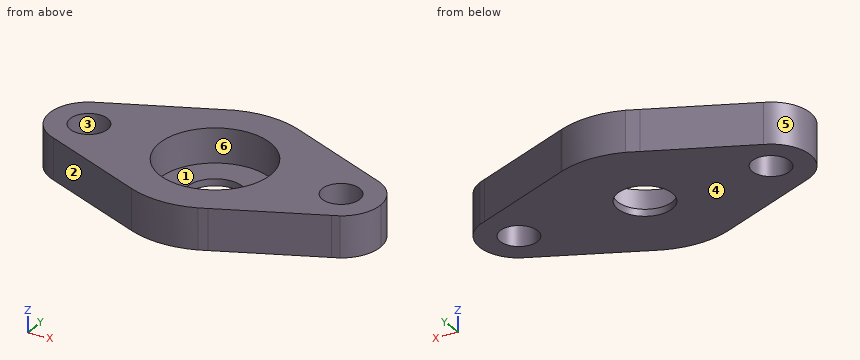
from build123d import *

# Parameters (mm, degrees)
F0_R     = 2.75
F0_R_2   = 4
F1_DEPTH = 6
F2_R     = 8.125
F2_R_2   = 4
F3_DEPTH = 5


# Not quite as in the source:
# - a feature names something its author has since deleted; it is built from what else it names


with BuildPart() as f1:
    # F0 (on Top) → F1 (new body)
    with BuildSketch(Plane.XY):
        with BuildLine():
            ThreePointArc((20.0822139412, 5.4502744952), (15.7589539647, 5.182392271), (12.8493150685, 1.9736013454))
            ThreePointArc((12.8493150685, 1.9736013454), (12.9622740268, 0.9896727008), (13, 0))
            ThreePointArc((13, 0), (12.9622740268, -0.9896727008), (12.8493150685, -1.9736013454))
            ThreePointArc((12.8493150685, -1.9736013454), (15.7262122641, -5.1665264409), (20.0130954241, -5.4730242577))
            Line((20.0130954241, -5.4730242577), (21.0412591059, -5.0270640143))
            ThreePointArc((21.0412591059, -5.0270640143), (23.2054131946, -2.9165699153), (24, 0))
            ThreePointArc((24, 0), (23.1883419046, 2.9453826972), (20.982511571, 5.0592371474))
            Line((20.982511571, 5.0592371474), (20.0822139412, 5.4502744952))
        make_face()
        with Locations((18.25, 0)):
            Circle(F0_R, mode=Mode.SUBTRACT)
        with BuildLine():
            Line((20.0822139412, 5.4502744952), (5.2758693561, 11.8812963323))
            ThreePointArc((5.2758693561, 11.8812963323), (10.328174214, 7.8948601891), (12.8493150685, 1.9736013454))
            ThreePointArc((12.8493150685, 1.9736013454), (15.7589539647, 5.182392271), (20.0822139412, 5.4502744952))
        make_face()
        with BuildLine():
            ThreePointArc((13, 0), (12.9622740268, 0.9896727008), (12.8493150685, 1.9736013454))
            ThreePointArc((12.8493150685, 1.9736013454), (12.5, 0), (12.8493150685, -1.9736013454))
            ThreePointArc((12.8493150685, -1.9736013454), (12.9622740268, -0.9896727008), (13, 0))
        make_face()
        with BuildLine():
            ThreePointArc((20.0130954241, -5.4730242577), (15.7262122641, -5.1665264409), (12.8493150685, -1.9736013454))
            ThreePointArc((12.8493150685, -1.9736013454), (10.4831727002, -7.6878534154), (5.7442785493, -11.6620437295))
            Line((5.7442785493, -11.6620437295), (20.0130954241, -5.4730242577))
        make_face()
        with BuildLine():
            Line((5.2758693561, 11.8812963323), (5.0818351063, 11.9655736157))
            ThreePointArc((5.0818351063, 11.9655736157), (0.4274688612, 12.9929700366), (-4.2843620194, 12.273721607))
            Line((-4.2843620194, 12.273721607), (-5.9821590265, 11.5418271249))
            ThreePointArc((-5.9821590265, 11.5418271249), (-10.5614317348, 7.5799841498), (-12.8493150685, 1.9736013454))
            ThreePointArc((-12.8493150685, 1.9736013454), (-12.588002192, 1.0021381252), (-12.5, 0))
            ThreePointArc((-12.5, 0), (-12.588002192, -1.0021381252), (-12.8493150685, -1.9736013454))
            ThreePointArc((-12.8493150685, -1.9736013454), (-10.2925346971, -7.9412675001), (-5.1687008476, -11.9283079918))
            ThreePointArc((-5.1687008476, -11.9283079918), (-0.3123803464, -12.9962463242), (4.589640736, -12.1628614197))
            Line((4.589640736, -12.1628614197), (5.7442785493, -11.6620437295))
            ThreePointArc((5.7442785493, -11.6620437295), (10.4831727002, -7.6878534154), (12.8493150685, -1.9736013454))
            ThreePointArc((12.8493150685, -1.9736013454), (12.5, 0), (12.8493150685, 1.9736013454))
            ThreePointArc((12.8493150685, 1.9736013454), (10.328174214, 7.8948601891), (5.2758693561, 11.8812963323))
        make_face()
        Circle(F0_R_2, mode=Mode.SUBTRACT)
        with BuildLine():
            ThreePointArc((-12.8493150685, -1.9736013454), (-13, 0), (-12.8493150685, 1.9736013454))
            ThreePointArc((-12.8493150685, 1.9736013454), (-15.8411768162, 5.2211177797), (-20.2535684755, 5.3896394466))
            ThreePointArc((-20.2535684755, 5.3896394466), (-23.9999641766, 0.020296977), (-20.2915681825, -5.3753603932))
            ThreePointArc((-20.2915681825, -5.3753603932), (-15.8596218943, -5.229588178), (-12.8493150685, -1.9736013454))
        make_face()
        with Locations((-18.25, 0)):
            Circle(F0_R, mode=Mode.SUBTRACT)
        with BuildLine():
            ThreePointArc((-12.5, 0), (-12.588002192, 1.0021381252), (-12.8493150685, 1.9736013454))
            ThreePointArc((-12.8493150685, 1.9736013454), (-13, 0), (-12.8493150685, -1.9736013454))
            ThreePointArc((-12.8493150685, -1.9736013454), (-12.588002192, -1.0021381252), (-12.5, 0))
        make_face()
        with BuildLine():
            ThreePointArc((-12.8493150685, 1.9736013454), (-10.5614317348, 7.5799841498), (-5.9821590265, 11.5418271249))
            Line((-5.9821590265, 11.5418271249), (-20.2535684755, 5.3896394466))
            ThreePointArc((-20.2535684755, 5.3896394466), (-15.8411768162, 5.2211177797), (-12.8493150685, 1.9736013454))
        make_face()
        with BuildLine():
            ThreePointArc((-5.1687008476, -11.9283079918), (-10.2925346971, -7.9412675001), (-12.8493150685, -1.9736013454))
            ThreePointArc((-12.8493150685, -1.9736013454), (-15.8596218943, -5.229588178), (-20.2915681825, -5.3753603932))
            Line((-20.2915681825, -5.3753603932), (-5.1687008476, -11.9283079918))
        make_face()
    extrude(amount=F1_DEPTH)

    # F2 (on face) → F3 (cut)
    with BuildSketch(Plane.XY.offset(6)):
        Circle(F2_R)
        Circle(F2_R_2, mode=Mode.SUBTRACT)
    extrude(amount=-F3_DEPTH, mode=Mode.SUBTRACT)


solid = f1.part
Geometry check sheet. Reference: the model listing, model coordinates, mm. Face numbers are marked on the shaded views. A direction names the side the tool comes from. Round coordinates to 2 decimals unless told otherwise and drop trailing zeros. Loops run counter-clockwise (first coordinate to the right, second up) from the corner with the lowest first, then second, coordinate; pieces in that order, holes last. Notation, with made-up numbers: (-28.5, 25) - (-17.5, 25) arc R31 ccw to (-17.5, 57) - close; hole circle Ø6 at (81, 63.25). An arc over 180 degrees is marked (long way). One line per question, with ' | ' between items. Start each with the question number.
1. Cross-section at C-C on y = 1.5. Record the cut outline in (x, z), then the cut area to 3 significant figures.
2. Cross-section at A-A on x = 0. Record the cut outline in (y, z) (3 decimals), then the cut area to 4 significant figures.
3. Tool access check on the marked faces 1 and 2. Record the directions out of +Z, -Z, +X, -X, +Y, -Y that give a thin tool (end or side, any length) a straight path to the whole face; none if there is none.
4. Draft check along X on the marked faces 3, 4, 5 and 6. Enter one of: released by +X, released by -X, zero draft, split by the parting line, or undercut.
5. Depth check by flat-ended pin: pin 1 (2 mm diameter, centred on x = 14.5, z = 1.5, fed in from -Y); pin 2 (8 mm diameter, centred on x = -1.5, y = 0, fed in from +Z); pin 3 (3 mm diameter, centred on x = -9.5, z = 3, fed in from +Y). Enter the tip coordinate at first touch or a pass-through.
6. Cross-section at D-D on x = -18.25. Record the cut outline in (y, z), then the cut area to 3 significant figures.
7. Scan lines: line 1 (Y direction, x = 0, z = 3.8) (3 decimals); line 2 (X direction, y = 1.75, z = 3.25); line 3 (X direction, y = -1.75, z = 0.8). Record each from-to range of solid material in increasing order. Write a range as [from, to].
8. Cross-section at B-B on z = 1.8. Record the cut outline in (x, y) (3 decimals).
Taken from the geometry:
1) outline: (-23.8, 0) - (-20.55, 0) - (-20.55, 6) - (-23.8, 6) - close; (-15.95, 0) - (-3.71, 0) - (-3.71, 1) - (-7.99, 1) - (-7.99, 6) - (-15.95, 6) - close; (3.71, 0) - (15.95, 0) - (15.95, 6) - (7.99, 6) - (7.99, 1) - (3.71, 1) - close; (20.55, 0) - (23.8, 0) - (23.8, 6) - (20.55, 6) - close | area: 143 mm²
2) outline: (-13, 0) - (-4, 0) - (-4, 1) - (-8.125, 1) - (-8.125, 6) - (-13, 6) - close; (4, 0) - (13, 0) - (13, 6) - (8.125, 6) - (8.125, 1) - (4, 1) - close | area: 66.75 mm²
3) face 1: +Z | face 2: +Z, -Z, -X, -Y
4) face 3: undercut | face 4: zero draft | face 5: released by -X | face 6: undercut
5) pin 1: y = -8.3 | pin 2: z = 1 | pin 3: y = 10.67
6) outline: (-6.26, 0) - (-2.75, 0) - (-2.75, 6) - (-6.26, 6) - close; (2.75, 0) - (6.25, 0) - (6.25, 6) - (2.75, 6) - close | area: 42.1 mm²
7) line 1: [-13, -8.125], [8.125, 13] | line 2: [-23.73, -20.37], [-16.13, -7.93], [7.93, 16.13], [20.37, 23.73] | line 3: [-23.73, -20.37], [-16.13, -3.6], [3.6, 16.13], [20.37, 23.73]
8) outline: (-20.292, -5.375) - (-5.169, -11.928) arc R13 ccw to (4.59, -12.163) - (21.041, -5.027) arc R5.75 ccw to (20.983, 5.059) - (5.082, 11.966) arc R13 ccw to (-4.284, 12.274) - (-20.254, 5.39) arc R5.75 ccw to start; hole circle Ø5.5 at (-18.25, 0); hole circle Ø16.25 at (0, 0); hole circle Ø5.5 at (18.25, 0)
